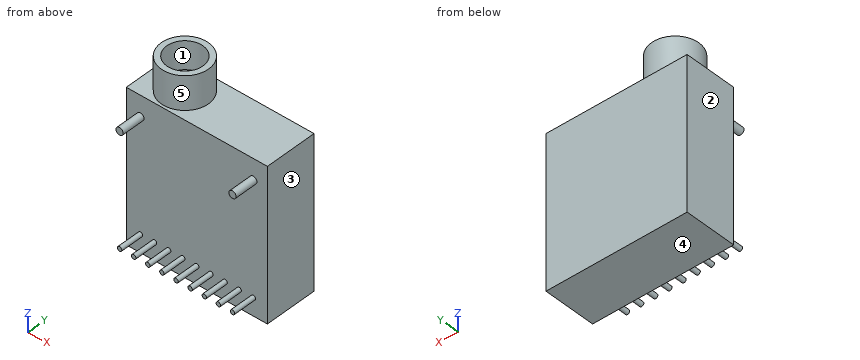
```python
from build123d import *

# Parameters (mm, degrees)
EXTRUDE_1_DEPTH      = 4.7
EXTRUDE_1_DEPTH_BACK = 4.7
SKETCH_1_W           = 25.4
SKETCH_1_H           = 27.2
SKETCH_2_R           = 4.25
EXTRUDE_2_DEPTH      = 6
SKETCH_3_R           = 3.25
CUT_EXTRUDE_1_DEPTH  = 5
SKETCH_4_R           = 0.65
SKETCH_4_R_2         = 0.4
EXTRUDE_3_DEPTH      = 4.2


with BuildPart() as part:
    # 草图1 → 凸台-拉伸1 (new, two sides: drawn at the far end of the back side and taken through both)
    with BuildSketch(Plane(origin=(0, 0, 0), x_dir=(1, 0, 0), z_dir=(0, 1, 0)).offset(-EXTRUDE_1_DEPTH_BACK)):
        Rectangle(SKETCH_1_W, SKETCH_1_H)
    extrude(amount=EXTRUDE_1_DEPTH + EXTRUDE_1_DEPTH_BACK)

    # 草图2 → 凸台-拉伸2 (add)
    with BuildSketch(Plane.XY.offset(13.6)):
        with Locations(Location((-6.35, 0, 0), (0, 0, 180))):
            Circle(SKETCH_2_R)
    extrude(amount=EXTRUDE_2_DEPTH)

    # 草图3 → 切除-拉伸1 (cut)
    with BuildSketch(Plane.XY.offset(19.6)):
        with Locations((-6.35, 0)):
            Circle(SKETCH_3_R)
    extrude(amount=-CUT_EXTRUDE_1_DEPTH, mode=Mode.SUBTRACT)

    # 草图4 → 凸台-拉伸3 (add)
    with BuildSketch(Plane.XZ.offset(4.7)):
        with Locations(Location((-10.16, 9.9, 0), (0, 0, 90))):
            Circle(SKETCH_4_R)
        with Locations(Location((10.16, 9.9, 0), (0, 0, 90))):
            Circle(SKETCH_4_R)
        with Locations(Location((-10.16, -10.4, 0), (0, 0, 90))):
            Circle(SKETCH_4_R_2)
        with Locations(Location((-7.62, -10.4, 0), (0, 0, 90))):
            Circle(SKETCH_4_R_2)
        with Locations(Location((-5.08, -10.4, 0), (0, 0, 90))):
            Circle(SKETCH_4_R_2)
        with Locations(Location((-2.54, -10.4, 0), (0, 0, 90))):
            Circle(SKETCH_4_R_2)
        with Locations(Location((0, -10.4, 0), (0, 0, 90))):
            Circle(SKETCH_4_R_2)
        with Locations(Location((2.54, -10.4, 0), (0, 0, 90))):
            Circle(SKETCH_4_R_2)
        with Locations(Location((5.08, -10.4, 0), (0, 0, 90))):
            Circle(SKETCH_4_R_2)
        with Locations(Location((7.62, -10.4, 0), (0, 0, 90))):
            Circle(SKETCH_4_R_2)
        with Locations(Location((10.16, -10.4, 0), (0, 0, 90))):
            Circle(SKETCH_4_R_2)
    extrude(amount=EXTRUDE_3_DEPTH)


solid = part.part
```
The model under review builds one solid part; all positions refer to its coordinate system, in mm. Face numbers are marked on the shaded views. A direction names the side the tool comes from. Give positions to 0.01 mm unless a question says otherwise; leave off trailing zeros. Write each loop counter-clockwise with the first axis right and the second up, starting at its lowest first coordinate (ties: lowest second). Pieces come first, ordered by that corner, then holes. Notation, with made-up numbers: M 62.5,52.25 L 106.5,52.25 A19 cw 106.5,69.25 Z; hole C 80,-36.5 d5. An arc over 180 degrees is marked long. Write item = value, one per line. Start each with the question number.
Q1. We need section B-B (z = 9.9). State the section outline as (x, y) points.
Q2. Clearance check with flat-ended pins moving along their axes: pin 1 (1.5 mm diameter, centred on x = 9.5, y = -2.5, fed in from +Z); pin 2 (5 mm diameter, centred on y = -6, z = 1.5, fed in from -X); pin 3 (4 mm diameter, centred on x = -6.35, y = 0, fed in from +Z); pin 4 (1.5 mm diameter, centred on x = 1.5, z = -4, fed in from -Y). State where each tip first meets the part, or that it passes through.
Q3. Mouldability with a two-part tool opening along X and no side actions: class the marked faces 1, 2 and 3 as released by +X, released by -X, zero draft, split by the parting line, or undercut.
Q4. We need section C-C (x = 5.08). State the section outline as (y, z) points.
Q5. We need section A-A (x = 10.16). State the section outline as (y, z) points.
Q6. For line 1 (Y direction, x = -6.35, z = 16.3); line 2 (Z direction, x = 5.25, y = -2.5); line 3 (Y direction, x = 4.5, z = 6.5), list the stretches that pass through material, from the lowest coordinate up.
Q7. We need section D-D (z = 14). State the section outline as (x, y) points.
Q8. Machinability: for the marked faces 4 and 5, which of the approach directions +Z, -Z, +X, -X, +Y, -Y give a long, thin tool a straight path to every point of the face, cutting with its end or side? Answer none if there is none.
Result set:
q1.outline = M -12.7,-4.7 L -10.81,-4.7 L -10.81,-8.9 L -9.51,-8.9 L -9.51,-4.7 L 9.51,-4.7 L 9.51,-8.9 L 10.81,-8.9 L 10.81,-4.7 L 12.7,-4.7 L 12.7,4.7 L -12.7,4.7 Z
q2.pin_1 = 13.6
q2.pin_2 = -12.7
q2.pin_3 = 14.6
q2.pin_4 = -4.7
q3.face_1 = undercut
q3.face_2 = released by -X
q3.face_3 = released by +X
q4.outline = M -8.9,-10.8 L -4.7,-10.8 L -4.7,-13.6 L 4.7,-13.6 L 4.7,13.6 L -4.7,13.6 L -4.7,-10 L -8.9,-10 Z
q5.outline = M -8.9,-10.8 L -4.7,-10.8 L -4.7,-13.6 L 4.7,-13.6 L 4.7,13.6 L -4.7,13.6 L -4.7,10.55 L -8.9,10.55 L -8.9,9.25 L -4.7,9.25 L -4.7,-10 L -8.9,-10 Z
q6.line_1 = -4.25 to -3.25, 3.25 to 4.25
q6.line_2 = -13.6 to 13.6
q6.line_3 = -4.7 to 4.7
q7.outline = C -6.35,0 d8.5
q8.face_4 = -Z, +X, -X, +Y, -Y
q8.face_5 = +Z
